Autodesk Inventor part; units mm, degrees
ref_plane "YZ Plane" through (0, 0, 0) normal (1, 0, 0) x (0, 1, 0)
ref_plane "XZ Plane" through (0, 0, 0) normal (0, 1, 0) x (-1, 0, 0)
ref_plane "XY Plane" through (0, 0, 0) normal (0, 0, 1) x (1, 0, 0)
sketch "Skizze1" plane through (0, 0, 0) normal (0, 0, 1) x (1, 0, 0)
  arc A0 (-28.686, -12.2792) -> (-28.686, 12.2792) centre (-1.314, 0) ccw
  line L0 (-28.686, -12.2792) -> (-28.686, 12.2792)
  line L1 (-29.486, 12.4492) -> (-29.486, -12.4492)
  arc A1 (-29.486, -12.4492) -> (-29.486, 12.4492) centre (-1.314, 0) ccw
  arc A2 (-30.686, -12.7) -> (-30.686, 12.7) centre (-1.314, 0) ccw
  line L2 (-30.686, 12.7) -> (-30.686, -12.7)
  point P0 (0, 0)
extrude "Extrusion1" add sketch "Skizze1" against normal blind 4 contours L2 A2
sketch "Skizze2" plane through (0, 0, 0) normal (0, 0, 1) x (1, 0, 0)
  line L0 (-30.686, 12.7) -> (-30.686, -12.7)
  arc A0 (-30.686, -12.7) -> (-30.686, 12.7) centre (-1.314, 0) ccw
  arc A1 (-28.686, -12.2792) -> (-28.686, 12.2792) centre (-1.314, 0) ccw
  line L1 (-28.686, -12.2792) -> (-28.686, 12.2792)
  point P0 (0, 0)
extrude "Extrusion2" add sketch "Skizze2" along normal blind 8
sketch "Skizze3" plane through (0, 0, 8) normal (0, 0, 1) x (1, 0, 0)
  arc A0 (-30.686, -12.7) -> (-30.686, 12.7) centre (-1.314, 0) ccw
  line L0 (-30.686, 12.7) -> (-30.686, -12.7)
  point P0 (0, 0)
extrude "Extrusion3" add sketch "Skizze3" along normal blind 2
sketch "Skizze4" plane through (0, 0, 10) normal (0, 0, 1) x (1, 0, 0)
  line L0 (12, -17.5) -> (-12, -17.5)
  line L1 (-12, 17.5) -> (12, 17.5)
  line L2 (-17.2, 8) -> (-17.2, -8)
  line L3 (-17.2, -8) -> (-12, -8)
  line L4 (-12, 8) -> (-17.2, 8)
  line L5 (-12, -17.5) -> (-12, -8)
  line L6 (-12, 8) -> (-12, 17.5)
  line L7 (17.2, -8) -> (17.2, 8)
  line L8 (-17.2, 8) -> (-17.2, -8)
  line L9 (-17.2, -8) -> (-12, -8)
  line L10 (12, -8) -> (17.2, -8)
  line L11 (17.2, 8) -> (12, 8)
  line L12 (-12, 8) -> (-17.2, 8)
  line L13 (12, 17.5) -> (12, 8)
  line L14 (12, -8) -> (12, -17.5)
  point P0 (0, 0)
  dimension "d32" = 34.4
extrude "Extrusion4" cut sketch "Skizze4" against normal blind 2
sketch "Skizze5" plane through (0, 0, 8) normal (0, 0, -1) x (-1, 0, 0)
  line L0 (17, 18) -> (-17, -18) construction
  line L1 (17, -18) -> (-17, 18) construction
  line L2 (-17.5, -18.5) -> (17.5, -18.5)
  line L3 (17.5, -18.5) -> (17.5, 18.5)
  line L4 (17.5, 18.5) -> (-17.5, 18.5)
  line L5 (-17.5, 18.5) -> (-17.5, -18.5)
  line L6 (18.5, -19.5) -> (-18.5, -19.5)
  line L7 (-18.5, -19.5) -> (-18.5, 19.5)
  line L8 (-18.5, 19.5) -> (18.5, 19.5)
  line L9 (18.5, 19.5) -> (18.5, -19.5)
  point P0 (0, 0)
  dimension "d17" = 1
extrude "Extrusion5" add sketch "Skizze5" along normal blind 3.9
sketch "Skizze7" plane through (-18.5, 19.5, 8) normal (0, 1, 0) x (1, 0, 0)
  line L0 (0, 0) -> (0, 3.9)
  line L1 (37, 0) -> (37, 3.9)
  line L2 (0, 0) -> (37, 0)
  line L3 (37, 0) -> (37, 2.475)
  line L4 (0, 2.475) -> (0, 0)
  circle A0 centre (24.7, 2.475) radius 0.875
  circle A1 centre (12.3, 2.475) radius 0.875
  point P0 (18.5, 8)
  dimension "d25" = 2.475
  dimension "d28" = 1.75
  dimension "d29" = 1.75
extrude "Extrusion6" cut sketch "Skizze7" against normal blind 40
sketch "Skizze8" plane through (0, 0, 10) normal (0, 0, 1) x (1, 0, 0)
  arc A0 (-30.686, -12.7) -> (-30.686, 12.7) centre (-1.314, 0) ccw
  line L0 (-30.686, 12.7) -> (-30.686, -12.7)
  line L1 (-12, 8) -> (-12, 17.5)
  line L2 (12, -17.5) -> (12, -8)
  line L3 (-12, 17.5) -> (12, 17.5)
  line L4 (12, 17.5) -> (12, -17.5)
  line L5 (12, -17.5) -> (-12, -17.5)
  line L6 (-12, -17.5) -> (-12, 17.5)
  point P0 (0, 0)
extrude "Extrusion7" add sketch "Skizze8" along normal blind 1
properties part number "Deckel"
Here's how the part is built. I have some questions about the finished solid (model axes, mm). A direction names the side the tool comes from. Give positions to 0.01 mm unless a question says otherwise; leave off trailing zeros. Write each loop counter-clockwise with the first axis right and the second up, starting at its lowest first coordinate (ties: lowest second). Pieces come first, ordered by that corner, then holes. Notation, with made-up numbers: (-17, 51.25) -> (8, 51.25) arc R7 ccw to (8, 60.25) -> close; hole circle Ø9 at (7.25, 38). An arc over 180 degrees is marked (long way). Write each question's results on one line, items separated by ' | '.
Item 1: Suppose I cut it at C-C on x = 27.5. Write out the boundary of the cut face in (y, z).
Output:
outline: (-13.92, -4) -> (-10.88, -4) -> (-10.88, 0) -> (-8.35, 0) -> (-8.35, 8) -> (8.35, 8) -> (8.35, 0) -> (10.88, 0) -> (10.88, -4) -> (13.92, -4) -> (13.92, 11) -> (-13.92, 11) -> close
Item 2: On a 3-axis mill with a long thin cutter (end or side, diameter ignored), from which of +Z, -Z, +X, -X, +Y, -Y can I reach the whole of each face in a straight line? I mean faces 1 (the face through (-5.365, -18.993, 5.262)), 2 (the face through (15, -8, 9)), 3 (the face through (0, 17.5, 9)). Say none if no direction works.
Output:
face 1: none | face 2: -Z | face 3: +Z, -Z
Item 3: We'd pull the mould along Z, two halves only. Please class faces 4 (the face through (-5.365, 19.007, 5.262)), 5 (the face through (15, 8, 9)), 6 (the face through (-30, -2, -4)): pulls with the +Z half, pulls with the -Z half, needs draft (parallel to the pull), parting line crosses it, or undercut.
Output:
face 4: undercut | face 5: needs draft | face 6: pulls with the -Z half
Item 4: For pin 1 Ø8 at (x, z) = (-4.5, 3.5) entering from -Y; pin 2 Ø5.5 at (x, y) = (14, -1.5) entering from -Z; pin 3 Ø2.5 at (x, z) = (6.2, 5.525) entering from -Y; pin 4 Ø1.5 at (y, z) = (0.5, 10) entering from +X, each with a flat end and sliding along its axis, tell me the tip position at first contact or that it passes through.
Output:
pin 1: stops at y = -32 | pin 2: stops at z = 10 | pin 3: stops at y = -31.38 | pin 4: stops at x = 30.69
Item 5: Suppose I cut it at D-D on z = -0.75. Write out the boundary of the cut face in (x, y).
Output:
outline: (-30.69, -12.7) arc R32 ccw (long way) to (-30.69, 12.7) -> close; hole (-29.49, -12.45) arc R30.8 ccw (long way) to (-29.49, 12.45) -> close
Item 6: If I drill on L1, parallel to Z at x = 6.2, y = 18.85; L2, parallel to X at y = 0, z = -1.65; L3, parallel to X at y = 0.5, z = 9.5, over which ranges is the centre line in solid material (lowest first)?
Output:
L1: z = 4.1 to 4.65, 6.4 to 11 | L2: x = -30.69 to -29.49, 29.49 to 30.69 | L3: x = -30.69 to -17.2, 17.2 to 30.68
Item 7: Suppose I cut it at A-A on y = 0. Write out the boundary of the cut face in (x, z).
Output:
outline: (-30.69, -4) -> (-29.49, -4) -> (-29.49, 0) -> (-28.69, 0) -> (-28.69, 8) -> (-18.5, 8) -> (-18.5, 4.1) -> (-17.5, 4.1) -> (-17.5, 8) -> (-17.2, 8) -> (-17.2, 10) -> (-12, 10) -> (-12, 11) -> (-30.69, 11) -> close; (12, 10) -> (17.2, 10) -> (17.2, 8) -> (17.5, 8) -> (17.5, 4.1) -> (18.5, 4.1) -> (18.5, 8) -> (28.69, 8) -> (28.69, 0) -> (29.49, 0) -> (29.49, -4) -> (30.69, -4) -> (30.69, 11) -> (12, 11) -> close
Item 8: Suppose I cut it at B-B on x = 6.2. Give the number of separate pieces and of enclosed holes in the cut face, plus the area to 3 significant figures.
Output:
separate pieces: 4 | enclosed holes: 0 | area: 129 mm^2
